from build123d import *

# Parameters (mm, degrees)
SKETCH2_R           = 9.75
SKETCH2_R_2         = 5.75
BOSS_EXTRUDE1_DEPTH = 2
SKETCH4_R           = 1.05
CUT_EXTRUDE1_DEPTH  = 3


with BuildPart() as part:
    # Sketch2 → Boss-Extrude1 (new body)
    with BuildSketch(Plane.XY):
        Circle(SKETCH2_R)
        Circle(SKETCH2_R_2, mode=Mode.SUBTRACT)
    extrude(amount=BOSS_EXTRUDE1_DEPTH)

    # Sketch4 → Cut-Extrude1 (cut, through all)
    with BuildSketch(Plane(origin=(0, 0, 0), x_dir=(-1, 0, 0), z_dir=(0, 0, -1))):
        with Locations((0, 7.5)):
            Circle(SKETCH4_R)
        with Locations((5.303300859, 5.303300859)):
            Circle(SKETCH4_R)
        with Locations((7.5, 0)):
            Circle(SKETCH4_R)
        with Locations((5.303300859, -5.303300859)):
            Circle(SKETCH4_R)
        with Locations((0, -7.5)):
            Circle(SKETCH4_R)
        with Locations((-5.303300859, -5.303300859)):
            Circle(SKETCH4_R)
        with Locations((-7.5, 0)):
            Circle(SKETCH4_R)
        with Locations((-5.303300859, 5.303300859)):
            Circle(SKETCH4_R)
    extrude(amount=-CUT_EXTRUDE1_DEPTH, mode=Mode.SUBTRACT)


solid = part.part
Design review of the part built by this model. Coordinates are the model's own, in mm. Coordinates: 2 decimals unless noted, no trailing zeros. Order: outer loops, then holes, each group sorted by start corner. A loop starts at its lowest first (then second) coordinate and runs counter-clockwise, first axis right, second up.
Item 1: The part is to be moulded in two halves that separate along X. For faces 1 (the cylindrical face through (5.53, 4.28, 0.99)), 2 (the cylindrical face through (-1.269, 9.667, 0.986)), 3 (the flat face through (4.2, -4.2, 0)), say which applies: pulls with the +X half, pulls with the -X half, needs draft (parallel to the pull), parting line crosses it, or undercut.
Item 2: For pin 1 Ø4 at (x, y) = (-6.5, 2.5) entering from -Z; pin 2 Ø1 at (y, z) = (4.5, 0.5) entering from -X; pin 3 Ø1 at (y, z) = (4, 1) entering from +X, all flat-tipped, find the tip position at first contact; note any pin that passes through.
Item 3: Take a section at B-B, the plane x = -1.75. Write out the cut boundary in (y, z).
Item 4: Take a section at C-C, the plane z = 0.65. Count the separate pieces of the cut face and the enclosed holes in it, then the cut area to 3 significant figures.
Item 5: For line 1 (Y direction, x = -5.25, z = 1.65); line 2 (Y direction, x = 6.25, z = 0.4); line 3 (Y direction, x = 0.75, z = 1.9), list the stretches that pass through material, from the lowest coordinate up.
Item 6: Take a section at D-D, the plane y = -7.5. Write out the cut boundary in (x, z), then the cut area to 3 significant figures.
Item 7: Take a section at A-A, the plane y = 0. Write out the cut boundary in (x, z).
The answers:
1. face 1: undercut
1. face 2: parting line crosses it
1. face 3: needs draft
2. pin 1: stops at z = 0
2. pin 2: stops at x = -8.89
2. pin 3: stops at x = 9.1
3. outline: (-9.59, 0) - (-5.48, 0) - (-5.48, 2) - (-9.59, 2) - close; (5.48, 0) - (9.59, 0) - (9.59, 2) - (5.48, 2) - close
4. separate pieces: 1
4. enclosed holes: 9
4. area: 167 mm2
5. line 1: y = -8.22 to -6.35, -4.25 to -2.35, 2.35 to 4.25, 6.35 to 8.22
5. line 2: y = -7.48 to -5.76, -4.85 to 4.85, 5.76 to 7.48
5. line 3: y = -9.72 to -8.23, -6.77 to -5.7, 5.7 to 6.77, 8.23 to 9.72
6. outline: (-6.23, 0) - (-1.05, 0) - (-1.05, 2) - (-6.23, 2) - close; (1.05, 0) - (6.23, 0) - (6.23, 2) - (1.05, 2) - close
6. area: 20.7 mm2
7. outline: (-9.75, 0) - (-8.55, 0) - (-8.55, 2) - (-9.75, 2) - close; (-6.45, 0) - (-5.75, 0) - (-5.75, 2) - (-6.45, 2) - close; (5.75, 0) - (6.45, 0) - (6.45, 2) - (5.75, 2) - close; (8.55, 0) - (9.75, 0) - (9.75, 2) - (8.55, 2) - close
